Work out the finished part from the listing and answer in its coordinate system (mm). Face numbers are marked on the shaded views. Coordinates: 2 decimals unless noted, no trailing zeros. Write each loop counter-clockwise with the first axis right and the second up, starting at its lowest first coordinate (ties: lowest second). Pieces come first, ordered by that corner, then holes. Notation, with made-up numbers: (6, -2) - (35, -2) arc R6 cw to (35, 6) - close; hole circle Ø4 at (-26.5, 36). An arc over 180 degrees is marked (long way). Use a Markdown table: item, result. Add a question column.
(1) The part is cut by section C-C, the plane z = -15. Give the vertices of the cut face in (x, y).
(2) For a pull along Z with two mould halves and no side action, classify the marked faces 1, 2, 3 and 4 as released by +Z, released by -Z, zero draft, split by the parting line, or undercut.
(3) The part is cut by section A-A, the plane y = 22. Give the vertices of the cut face in (x, z).
(4) The part is cut by section B-B, the plane x = -22.5. Give the vertices of the cut face in (y, z).
(5) Find the intervals of material crossed by line 1 (Z direction, x = -46, y = 52); line 2 (X direction, y = 24, z = -8); line 3 (Y direction, x = 14, z = -25.5), in increasing order. Write a range as from..to.
(6) Given pin 1 Ø1.5 at (x, z) = (-65.5, -32) entering from -Y; pin 2 Ø1.5 at (y, z) = (70.5, -31.5) entering from +X; pin 3 Ø23 at (x, z) = (-26.5, -11.5) entering from -Y, each flat-ended and moving along its own axis, determine where each tip first touches the part or whether it passes through.
from build123d import *

# Parameters (mm, degrees)
F0_W     = 152.4
F0_H     = 50.8
F1_DEPTH = 76.2
F2_W     = 147.48656
F2_H     = 45.76164
F3_DEPTH = 71.12
F4_W     = 5.08
F4_H     = 5.080001
F4_H_2   = 5.08
F5_DEPTH = 5.08
F6_W     = 5.08
F6_H     = 5.08
F7_DEPTH = 5.08


with BuildPart() as f1:
    # F0 (on Front) → F1 (new body)
    with BuildSketch(Plane.XZ):
        with Locations((5.538031, -3.279099)):
            Rectangle(F0_W, F0_H)
    extrude(amount=-F1_DEPTH)

    # F2 (on Front) → F3 (cut)
    with BuildSketch(Plane.XZ):
        with Locations((5.683769, -3.497704)):
            Rectangle(F2_W, F2_H)
    extrude(amount=-F3_DEPTH, mode=Mode.SUBTRACT)

    # F4 (on face) → F5 (join)
    with BuildSketch(Plane(origin=(0, 0, -28.679099), x_dir=(1, 0, 0), z_dir=(0, 0, -1))):
        with Locations((-65.581969, -5.08)):
            Rectangle(F4_W, F4_H)
        with Locations((76.658031, -5.08)):
            Rectangle(F4_W, F4_H)
        with Locations((76.658031, -71.12)):
            Rectangle(F4_W, F4_H)
        with Locations((-65.581969, -71.12)):
            Rectangle(F4_W, F4_H_2)
    extrude(amount=F5_DEPTH)

    # F6 (on face) → F7 (cut)
    with BuildSketch(Plane.XY.offset(22.120901)):
        with Locations((-65.581969, 71.12)):
            Rectangle(F6_W, F6_H)
        with Locations((-65.581969, 5.08)):
            Rectangle(F6_W, F6_H)
        with Locations((76.658031, 71.12)):
            Rectangle(F6_W, F6_H)
        with Locations((76.658031, 5.08)):
            Rectangle(F6_W, F6_H)
    extrude(amount=-F7_DEPTH, mode=Mode.SUBTRACT)


solid = f1.part
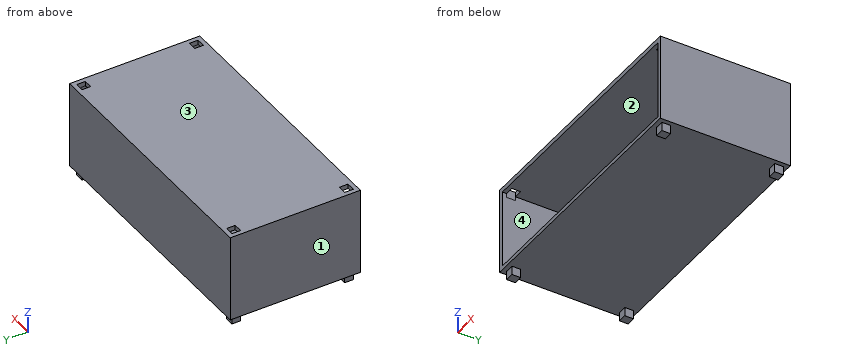
Model answer:
| question | item | result |
|---|---|---|
| 1 | outline | (-70.66, 0) - (-68.06, 0) - (-68.06, 71.12) - (79.43, 71.12) - (79.43, 0) - (81.74, 0) - (81.74, 76.2) - (-70.66, 76.2) - close |
| 2 | face 1 | zero draft |
| 2 | face 2 | undercut |
| 2 | face 3 | released by +Z |
| 2 | face 4 | undercut |
| 3 | outline | (-70.66, -28.68) - (81.74, -28.68) - (81.74, 22.12) - (-70.66, 22.12) - close; hole (-68.06, -26.38) - (79.43, -26.38) - (79.43, 19.38) - (-68.06, 19.38) - close |
| 4 | outline | (0, -28.68) - (76.2, -28.68) - (76.2, 22.12) - (0, 22.12) - (0, 19.38) - (71.12, 19.38) - (71.12, -26.38) - (0, -26.38) - close |
| 5 | line 1 | -28.68..-26.38, 19.38..22.12 |
| 5 | line 2 | -70.66..-68.06, 79.43..81.74 |
| 5 | line 3 | 71.12..76.2 |
| 6 | pin 1 | y = 2.54 |
| 6 | pin 2 | x = 79.2 |
| 6 | pin 3 | y = 71.12 |
